The model under review builds one solid part; all positions refer to its coordinate system, in mm. Face numbers are marked on the shaded views. A direction names the side the tool comes from. Round coordinates to 2 decimals unless told otherwise and drop trailing zeros. Write each loop counter-clockwise with the first axis right and the second up, starting at its lowest first coordinate (ties: lowest second). Pieces come first, ordered by that corner, then holes. Notation, with made-up numbers: M 45.5,-22 L 68.5,-22 A22 cw 68.5,8 Z; hole C 71.5,18 d9. An arc over 180 degrees is marked long. One line per item, written item: value. Start each with the question number.
1) Wall thickness on probe 1 along Z at (x, y) = (38, -48); probe 2 along Y at (x, z) = (42, -27); probe 3 along Z at (x, y) = (7.5, -4.5): over which ranges is each line inside the solid? List them lowest first.
2) For P1, Ø8, axis at x = 37.77, y = -31.42, coming from the -Z side; P2, Ø7, axis at x = 13.03, y = -6.68, coming from the +Z side; P3, Ø6, axis at x = 7.5, z = -35, coming from the +Y side, all flat-tipped, find the tip position at first contact; note any pin that passes through.
3) Tool access review of the marked faces 1 and 2: name each direction out of +Z, -Z, +X, -X, +Y, -Y from which nothing blocks a thin tool from reaching the whole face with its end or side.
4) Take a section at A-A, the plane y = -19.05. Write out the cut boundary in (x, z), and give its area (3 significant figures).
5) Mouldability with a two-part tool opening along Y and no side actions: class the marked faces 3, 4 and 5 as +Y half, -Y half, draft (parallel to the pull), parting line (faces both ways), or undercut.
6) Take a section at D-D, the plane x = 46.5. Write out the cut boundary in (y, z).
7) Take a section at C-C, the plane z = -23. Write out the cut boundary in (x, y), and give its area (3 significant figures).
8) Take a section at B-B, the plane x = 25.4. Write out the cut boundary in (y, z).
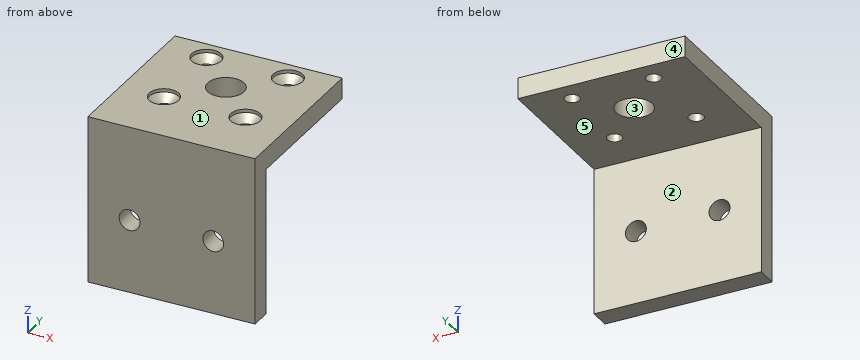
from build123d import *

# Parameters (mm, degrees)
BOSS_EXTRUDE1_DEPTH          = 50.8
CUT_EXTRUDE1_REACH           = 86.481
SKETCH2_R                    = 2.25
SKETCH2_R_2                  = 5.5
CUT_EXTRUDE2_REACH           = 82.822
SKETCH4_R                    = 3.175
CSK_FOR_M4_SFHCS1_AT_2_COUNT = 2
CSK_FOR_M4_SFHCS1_AT_2_PITCH = 24.748737342
CSK_FOR_M4_SFHCS1_AT_3_COUNT = 2
CSK_FOR_M4_SFHCS1_AT_3_PITCH = 35
CSK_FOR_M4_SFHCS1_AT_4_COUNT = 2
CSK_FOR_M4_SFHCS1_AT_4_PITCH = 24.748737342


with BuildPart() as part:
    # Sketch1 → Boss-Extrude1 (new body)
    with BuildSketch(Plane(origin=(0, 0, 0), x_dir=(0, 0, -1), z_dir=(1, 0, 0))):
        Polygon((0, 0), (0, -44.45), (44.45, -44.45), (44.45, -50.8), (-6.35, -50.8), (-6.35, 0), align=None)
    extrude(amount=BOSS_EXTRUDE1_DEPTH)

    # Sketch2 → Cut-Extrude1 (cut, up to next)
    with BuildSketch(Plane(origin=(0, 0, 0), x_dir=(-1, 0, 0), z_dir=(0, 0, -1)), mode=Mode.PRIVATE) as cut_extrude1_sk1:
        with Locations(Location((-13.025631329, -6.675631329, 0), (0, 0, 90))):
            Circle(SKETCH2_R)
    cut_extrude1_tool1 = extrude(cut_extrude1_sk1.sketch, amount=-CUT_EXTRUDE1_REACH, mode=Mode.PRIVATE) & part.part
    # Sketch2 → Cut-Extrude1 (cut, up to next)
    with BuildSketch(Plane(origin=(0, 0, 0), x_dir=(-1, 0, 0), z_dir=(0, 0, -1)), mode=Mode.PRIVATE) as cut_extrude1_sk2:
        with Locations(Location((-13.025631329, -31.424368671, 0), (0, 0, 90))):
            Circle(SKETCH2_R)
    cut_extrude1_tool2 = extrude(cut_extrude1_sk2.sketch, amount=-CUT_EXTRUDE1_REACH, mode=Mode.PRIVATE) & part.part
    # Sketch2 → Cut-Extrude1 (cut, up to next)
    with BuildSketch(Plane(origin=(0, 0, 0), x_dir=(-1, 0, 0), z_dir=(0, 0, -1)), mode=Mode.PRIVATE) as cut_extrude1_sk3:
        with Locations(Location((-37.774368671, -31.424368671, 0), (0, 0, 90))):
            Circle(SKETCH2_R)
    cut_extrude1_tool3 = extrude(cut_extrude1_sk3.sketch, amount=-CUT_EXTRUDE1_REACH, mode=Mode.PRIVATE) & part.part
    # Sketch2 → Cut-Extrude1 (cut, up to next)
    with BuildSketch(Plane(origin=(0, 0, 0), x_dir=(-1, 0, 0), z_dir=(0, 0, -1)), mode=Mode.PRIVATE) as cut_extrude1_sk4:
        with Locations(Location((-37.774368671, -6.675631329, 0), (0, 0, 90))):
            Circle(SKETCH2_R)
    cut_extrude1_tool4 = extrude(cut_extrude1_sk4.sketch, amount=-CUT_EXTRUDE1_REACH, mode=Mode.PRIVATE) & part.part
    # Sketch2 → Cut-Extrude1 (cut, up to next)
    with BuildSketch(Plane(origin=(0, 0, 0), x_dir=(-1, 0, 0), z_dir=(0, 0, -1)), mode=Mode.PRIVATE) as cut_extrude1_sk5:
        with Locations(Location((-25.4, -19.05, 0), (0, 0, 90))):
            Circle(SKETCH2_R_2)
    cut_extrude1_tool5 = extrude(cut_extrude1_sk5.sketch, amount=-CUT_EXTRUDE1_REACH, mode=Mode.PRIVATE) & part.part
    add(cut_extrude1_tool1.solids().sort_by_distance((13.025631, -6.675631, 0))[0], mode=Mode.SUBTRACT)
    add(cut_extrude1_tool2.solids().sort_by_distance((13.025631, -31.424369, 0))[0], mode=Mode.SUBTRACT)
    add(cut_extrude1_tool3.solids().sort_by_distance((37.774369, -31.424369, 0))[0], mode=Mode.SUBTRACT)
    add(cut_extrude1_tool4.solids().sort_by_distance((37.774369, -6.675631, 0))[0], mode=Mode.SUBTRACT)
    add(cut_extrude1_tool5.solids().sort_by_distance((25.4, -19.05, 0))[0], mode=Mode.SUBTRACT)

    # Sketch4 → Cut-Extrude2 (cut, up to next)
    with BuildSketch(Plane(origin=(0, -44.45, 0), x_dir=(1, 0, 0), z_dir=(0, 1, 0)), mode=Mode.PRIVATE) as cut_extrude2_sk1:
        with Locations(Location((12.7, 22.225, 0), (0, 0, 270))):
            Circle(SKETCH4_R)
    cut_extrude2_tool1 = extrude(cut_extrude2_sk1.sketch, amount=-CUT_EXTRUDE2_REACH, mode=Mode.PRIVATE) & part.part
    # Sketch4 → Cut-Extrude2 (cut, up to next)
    with BuildSketch(Plane(origin=(0, -44.45, 0), x_dir=(1, 0, 0), z_dir=(0, 1, 0)), mode=Mode.PRIVATE) as cut_extrude2_sk2:
        with Locations(Location((38.1, 22.225, 0), (0, 0, 270))):
            Circle(SKETCH4_R)
    cut_extrude2_tool2 = extrude(cut_extrude2_sk2.sketch, amount=-CUT_EXTRUDE2_REACH, mode=Mode.PRIVATE) & part.part
    add(cut_extrude2_tool1.solids().sort_by_distance((12.7, -44.45, -22.225))[0], mode=Mode.SUBTRACT)
    add(cut_extrude2_tool2.solids().sort_by_distance((38.1, -44.45, -22.225))[0], mode=Mode.SUBTRACT)

    # Sketch5 → CSK for M4 SFHCS1 (revolve, cut)
    with BuildSketch(Plane(origin=(13.025631329, -6.675631329, 6.35), x_dir=(0, -1, 0), z_dir=(1, 0, 0))):
        Polygon((0, 0), (0, 50.8), (2.15, 50.8), (2.15, 3.346), (4.48, 1.016), (4.48, 0), align=None)
    csk_for_m4_sfhcs1 = revolve(axis=Axis((13.025631329, -6.675631329, 12.7), (0, 0, -1)), mode=Mode.SUBTRACT)

    # CSK for M4 SFHCS1 at 2: CSK for M4 SFHCS1 ×2
    with Locations(*[(i * CSK_FOR_M4_SFHCS1_AT_2_PITCH, 0, 0) for i in range(1, CSK_FOR_M4_SFHCS1_AT_2_COUNT)]):
        add(csk_for_m4_sfhcs1, mode=Mode.SUBTRACT)

    # CSK for M4 SFHCS1 at 3: CSK for M4 SFHCS1 ×2
    with Locations(*[Vector(0.7071067811865426, -0.7071067811865525, 0) * (i * CSK_FOR_M4_SFHCS1_AT_3_PITCH) for i in range(1, CSK_FOR_M4_SFHCS1_AT_3_COUNT)]):
        add(csk_for_m4_sfhcs1, mode=Mode.SUBTRACT)

    # CSK for M4 SFHCS1 at 4: CSK for M4 SFHCS1 ×2
    with Locations(*[(0, -i * CSK_FOR_M4_SFHCS1_AT_4_PITCH, 0) for i in range(1, CSK_FOR_M4_SFHCS1_AT_4_COUNT)]):
        add(csk_for_m4_sfhcs1, mode=Mode.SUBTRACT)


solid = part.part
Checked values:
1. probe 1: z = -44.45 to -25.4, -19.05 to 6.35
1. probe 2: y = -50.8 to -44.45
1. probe 3: z = 0 to 6.35
2. P1: stops at z = 0
2. P2: stops at z = 4.36
2. P3: stops at y = -44.45
3. face 1: +Z, +X, -X, +Y, -Y
3. face 2: -Z, +X, -X, +Y
4. outline: M 0,0 L 19.9,0 L 19.9,6.35 L 0,6.35 Z; M 30.9,0 L 50.8,0 L 50.8,6.35 L 30.9,6.35 Z
4. area: 253 mm2
5. face 3: undercut
5. face 4: +Y half
5. face 5: draft
6. outline: M -50.8,-44.45 L -44.45,-44.45 L -44.45,0 L 0,0 L 0,6.35 L -50.8,6.35 Z
7. outline: M 0,-50.8 L 9.62,-50.8 L 9.62,-44.45 L 0,-44.45 Z; M 15.78,-50.8 L 35.02,-50.8 L 35.02,-44.45 L 15.78,-44.45 Z; M 41.18,-50.8 L 50.8,-50.8 L 50.8,-44.45 L 41.18,-44.45 Z
7. area: 244 mm2
8. outline: M -50.8,-44.45 L -44.45,-44.45 L -44.45,0 L -24.55,0 L -24.55,6.35 L -50.8,6.35 Z; M -13.55,0 L 0,0 L 0,6.35 L -13.55,6.35 Z
